Geometry check sheet. Reference: the model listing, model coordinates, mm. A direction names the side the tool comes from. Give positions to 0.01 mm unless a question says otherwise; leave off trailing zeros. Order: outer loops, then holes, each group sorted by start corner. A loop starts at its lowest first (then second) coordinate and runs counter-clockwise, first axis right, second up.
```python
from build123d import *

# Parameters (mm, degrees)
SKETCH1_W           = 36
SKETCH1_H           = 15
SKETCH1_R           = 1.7
SKETCH1_R_2         = 1.65
SKETCH1_R_3         = 1.6
SKETCH1_R_4         = 1.5
SKETCH1_R_5         = 1.55
BOSS_EXTRUDE1_DEPTH = 10
FILLET2_R           = 3
CHAMFER2_SIZE       = 3
SKETCH3_W           = 10
SKETCH3_H           = 6
CUT_EXTRUDE1_DEPTH  = 10


with BuildPart() as part:
    # Sketch1 → Boss-Extrude1 (new body)
    with BuildSketch(Plane.XY):
        with Locations((0, -2.5)):
            Rectangle(SKETCH1_W, SKETCH1_H)
        with Locations((12.3, 0)):
            Circle(SKETCH1_R, mode=Mode.SUBTRACT)
        with Locations((5.95, 0)):
            Circle(SKETCH1_R_2, mode=Mode.SUBTRACT)
        with Locations((-0.3, 0)):
            Circle(SKETCH1_R_3, mode=Mode.SUBTRACT)
        with Locations((-12.5, 0)):
            Circle(SKETCH1_R_4, mode=Mode.SUBTRACT)
        with Locations((-6.45, 0)):
            Circle(SKETCH1_R_5, mode=Mode.SUBTRACT)
    extrude(amount=BOSS_EXTRUDE1_DEPTH)

    # Fillet2
    fillet2_edges = [part.edges().sort_by_distance(p)[0] for p in [
        (-18, 5, 5),
    ]]
    fillet(fillet2_edges, radius=FILLET2_R)

    # Chamfer2
    chamfer2_edges = [part.edges().sort_by_distance(p)[0] for p in [
        (18, 5, 5),
    ]]
    chamfer(chamfer2_edges, length=CHAMFER2_SIZE)

    # Sketch3 → Cut-Extrude1 (cut)
    with BuildSketch(Plane.XY.offset(10)):
        with Locations((0, -10)):
            Rectangle(SKETCH3_W, SKETCH3_H)
    extrude(amount=-CUT_EXTRUDE1_DEPTH, mode=Mode.SUBTRACT)


solid = part.part
```
Q1. Access from +Z, -Z, +X, -X, +Y, -Y to the whole of each face (thin tool, end or side, straight path). Record for faces 4 (the face through (0, -7, 5)), 5 (the face through (11, -10, 5)).
Q2. Release check for a two-part mould opening along X. For faces 1 (the face through (0, -2, 10)), 2 (the face through (18, -4, 5)), 3 (the face through (10.95, -1.03, 4.93)) record: pulls with the +X half, pulls with the -X half, needs draft (parallel to the pull), parting line crosses it, or undercut.
Q3. Cross-section at D-D, the plane z = 1.5. Record the boundary of the cut face in (x, y), and give its area (3 significant figures).
Q4. Thickness scan on L1, parallel to X at y = -8.5, z = 7.25; L2, parallel to Y at x = 5.95, z = 7; L3, parallel to Y at x = 12.3, z = 2.75. Record the ranges inside material, lowest first.
Q5. Gauge pin test, flat end, axial feed: P1, Ø4, axis at x = -6.45, y = 0, coming from the -Z side. Record the tip position at first contact, or that the pin passes through.
Q6. Cross-section at B-B, the plane y = 0. Record the boundary of the cut face in (x, z), and give its area (3 significant figures).
Q7. Cross-section at A-A, the plane x = -0.3. Record the boundary of the cut face in (y, z), and give its area (3 significant figures).
Q8. Cross-section at C-C, the plane y = -8.25. Record the boundary of the cut face in (x, z).
Answers follow:
1. face 4: +Z, -Z, -Y
1. face 5: +Z, -Z, +X, -X, -Y
2. face 1: needs draft
2. face 2: pulls with the +X half
2. face 3: undercut
3. outline: (-18, -10) - (-5, -10) - (-5, -7) - (5, -7) - (5, -10) - (18, -10) - (18, 2) - (15, 5) - (-15, 5) arc R3 ccw to (-18, 2) - close; hole circle Ø3 at (-12.5, 0); hole circle Ø3.1 at (-6.45, 0); hole circle Ø3.2 at (-0.3, 0); hole circle Ø3.3 at (5.95, 0); hole circle Ø3.4 at (12.3, 0)
3. area: 463 mm2
4. L1: x = -18 to -5, 5 to 18
4. L2: y = -10 to -1.65, 1.65 to 5
4. L3: y = -10 to -1.7, 1.7 to 5
5. P1: stops at z = 0
6. outline: (-18, 0) - (-14, 0) - (-14, 10) - (-18, 10) - close; (-11, 0) - (-8, 0) - (-8, 10) - (-11, 10) - close; (-4.9, 0) - (-1.9, 0) - (-1.9, 10) - (-4.9, 10) - close; (1.3, 0) - (4.3, 0) - (4.3, 10) - (1.3, 10) - close; (7.6, 0) - (10.6, 0) - (10.6, 10) - (7.6, 10) - close; (14, 0) - (18, 0) - (18, 10) - (14, 10) - close
6. area: 200 mm2
7. outline: (-7, 0) - (-1.6, 0) - (-1.6, 10) - (-7, 10) - close; (1.6, 0) - (5, 0) - (5, 10) - (1.6, 10) - close
7. area: 88.0 mm2
8. outline: (-18, 0) - (-5, 0) - (-5, 10) - (-18, 10) - close; (5, 0) - (18, 0) - (18, 10) - (5, 10) - close
